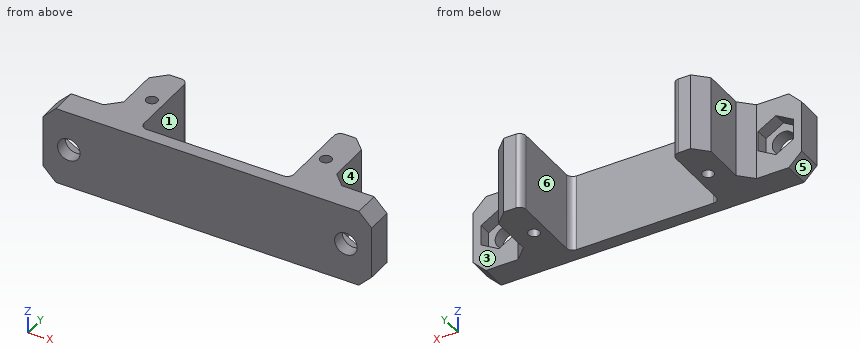
from build123d import *

# Parameters (mm, degrees)
F0_R     = 0.875
F1_DEPTH = 12
F2_SIZE  = 2
F3_R     = 1.75
F4_DEPTH = 4
F5_DEPTH = 2
F6_R     = 1


with BuildPart() as f1:
    # F0 (on Top) → F1 (new body)
    with BuildSketch(Plane.XY):
        Polygon((11.625, -5.25), (-11.625, -5.25), (-16.5, -5.25), (-16.5, -7.25), (16.5, -7.25), (16.5, -5.25), align=None)
        Polygon((-16.5, -5.25), (-16.5, -3.25), (-25.5, -3.25), (-25.5, -7.25), (-16.5, -7.25), align=None)
        Polygon((25.5, -3.25), (16.5, -3.25), (16.5, -5.25), (16.5, -7.25), (25.5, -7.25), align=None)
        Polygon((-11.625, 7.25), (-16.5, 7.25), (-16.5, -3.25), (-16.5, -5.25), (-11.625, -5.25), align=None)
        with Locations((-13.5, 1)):
            Circle(F0_R, mode=Mode.SUBTRACT)
        Polygon((16.5, 7.25), (11.625, 7.25), (11.625, -5.25), (16.5, -5.25), (16.5, -3.25), align=None)
        with Locations((13.5, 1)):
            Circle(F0_R, mode=Mode.SUBTRACT)
    extrude(amount=F1_DEPTH)

    # F2
    f2_edges = [f1.edges().sort_by_distance(p)[0] for p in [
        (-16.5, -3.25, 6),
        (16.5, -3.25, 6),
        (25.5, -5.25, 12),
        (25.5, -5.25, 0),
        (-25.5, -5.25, 12),
        (-25.5, -5.25, 0),
        (16.5, 7.25, 6),
        (-16.5, 7.25, 6),
    ]]
    chamfer(f2_edges, length=F2_SIZE)

    # F3 (on face) → F4 (cut, through all)
    with BuildSketch(Plane(origin=(0, -3.25, 0), x_dir=(-1, 0, 0), z_dir=(0, 1, 0))):
        with Locations((21.5, 6)):
            Circle(F3_R)
        with Locations((-21.5, 6)):
            Circle(F3_R)
    extrude(amount=-F4_DEPTH, mode=Mode.SUBTRACT)

    # F3 (on face) → F5 (cut)
    with BuildSketch(Plane(origin=(0, -3.25, 0), x_dir=(-1, 0, 0), z_dir=(0, 1, 0))):
        Polygon((-18.75, 4.4122867597), (-18.75, 7.5877132403), (-21.5, 9.1754264805), (-24.25, 7.5877132403), (-24.25, 4.4122867597), (-21.5, 2.8245735195), align=None)
        with Locations((-21.5, 6)):
            Circle(F3_R, mode=Mode.SUBTRACT)
        Polygon((18.75, 7.5877132403), (18.75, 4.4122867597), (21.5, 2.8245735195), (24.25, 4.4122867597), (24.25, 7.5877132403), (21.5, 9.1754264805), align=None)
        with Locations((21.5, 6)):
            Circle(F3_R, mode=Mode.SUBTRACT)
    extrude(amount=-F5_DEPTH, mode=Mode.SUBTRACT)

    # F6
    f6_edges = [f1.edges().sort_by_distance(p)[0] for p in [
        (11.625, -5.25, 6),
        (-11.625, -5.25, 6),
        (-11.625, 7.25, 6),
        (11.625, 7.25, 6),
    ]]
    fillet(f6_edges, radius=F6_R)


solid = f1.part
The listing builds one solid part. Answer for the finished solid, in the listing's coordinates (mm). Face numbers are marked on the shaded views. A direction names the side the tool comes from. Give positions to 0.01 mm unless a question says otherwise; leave off trailing zeros. Write each loop counter-clockwise with the first axis right and the second up, starting at its lowest first coordinate (ties: lowest second). Pieces come first, ordered by that corner, then holes.
Item 1: Section A-A, the plane y = -3.75 is taken. Write down the section's boundary in (x, z) (3 decimals), plus the area to 3 significant figures.
Item 2: Section B-B, the plane x = 13.5 is taken. Write down the section's boundary in (y, z) (3 decimals), plus the area to 3 significant figures.
Item 3: Determine the mould class of the marked faces 4, 5 and 6 for opening direction X: released by +X, released by -X, zero draft, split by the parting line, or undercut.
Item 4: Flat-ended cylindrical pins translate along their axes: P1, Ø5, axis at y = 4.5, z = 3, coming from the +X side; P2, Ø1, axis at x = -17.5, z = 5.5, coming from the +Y side; P3, Ø5, axis at x = 18.5, z = 1.5, coming from the +Y side. Find the tip coordinate at first contact, or state that the pin passes through.
Item 5: Find the intervals of material crossed by line 1 along Y through (x, z) = (-13.5, 4) (3 decimals); line 2 along X through (y, z) = (3.5, 3.5) (3 decimals); line 3 along X through (y, z) = (1.25, 10.75) (3 decimals), in increasing order.
Item 6: Section C-C, the plane y = 1 is taken. Write down the section's boundary in (x, z) (3 decimals), plus the area to 3 significant figures.
Item 7: Section D-D, the plane y = 4.75 is taken. Write down the section's boundary in (x, z) (3 decimals).
Item 8: Which of the six approach directions +Z, -Z, +X, -X, +Y, -Y give full straight-line access (tool end or side, diameter ignored) to the marked faces 1, 2 and 3?
Completed:
1. outline: (-25.5, 2) - (-23.5, 0) - (-11.625, 0) - (-11.625, 12) - (-23.5, 12) - (-25.5, 10) - close; (11.625, 0) - (23.5, 0) - (25.5, 2) - (25.5, 10) - (23.5, 12) - (11.625, 12) - close; hole (-24.25, 4.412) - (-21.5, 2.825) - (-18.75, 4.412) - (-18.75, 7.588) - (-21.5, 9.175) - (-24.25, 7.588) - close; hole (18.75, 4.412) - (21.5, 2.825) - (24.25, 4.412) - (24.25, 7.588) - (21.5, 9.175) - (18.75, 7.588) - close
1. area: 273 mm2
2. outline: (-7.25, 0) - (0.125, 0) - (0.125, 12) - (-7.25, 12) - close; (1.875, 0) - (7.25, 0) - (7.25, 12) - (1.875, 12) - close
2. area: 153 mm2
3. face 4: released by +X
3. face 5: released by -X
3. face 6: undercut
4. P1: stops at x = 16.5
4. P2: stops at y = -1.75
4. P3: stops at y = 5.75
5. line 1: y = -7.25 to 0.125, 1.875 to 7.25
5. line 2: x = -16.5 to -11.625, 11.625 to 16.5
5. line 3: x = -16.5 to -14.339, -12.661 to -11.625, 11.625 to 12.661, 14.339 to 16.5
6. outline: (-16.5, 0) - (-14.375, 0) - (-14.375, 12) - (-16.5, 12) - close; (-12.625, 0) - (-11.625, 0) - (-11.625, 12) - (-12.625, 12) - close; (11.625, 0) - (12.625, 0) - (12.625, 12) - (11.625, 12) - close; (14.375, 0) - (16.5, 0) - (16.5, 12) - (14.375, 12) - close
6. area: 75.0 mm2
7. outline: (-16.5, 0) - (-11.625, 0) - (-11.625, 12) - (-16.5, 12) - close; (11.625, 0) - (16.5, 0) - (16.5, 12) - (11.625, 12) - close
8. face 1: +Z, -Z, +Y
8. face 2: +Z, -Z, -X, +Y
8. face 3: +Z, -Z, +X, +Y
